```python
from build123d import *
from build123d.topology import SkipClean

# Parameters (mm, degrees)
BOSS_EXTRUDE1_DEPTH           = 2
BOSS_EXTRUDE2_DEPTH           = 80
SKETCH3_R                     = 2.5
BOSS_EXTRUDE3_DEPTH           = 8
BOSS_EXTRUDE3_DRAFT           = 3
BOSS_EXTRUDE3_PROFILE_2_DEPTH = 8
BOSS_EXTRUDE3_PROFILE_2_DRAFT = 3
SHELL2_START                  = 1
SHELL2_OUTLINE_R              = 9
SHELL2_DEPTH                  = 80
CUT_EXTRUDE1_DEPTH            = 93.332280474
BOSS_EXTRUDE4_DEPTH           = 5
BOSS_EXTRUDE5_DEPTH           = 5


with BuildPart() as part:
    # Sketch1 → Boss-Extrude1 (new body)
    with BuildSketch(Plane(origin=(0, 0, 0), x_dir=(1, 0, 0), z_dir=(0, 1, 0))):
        with BuildLine():
            Line((-15, -12.5), (15, -12.5))
            ThreePointArc((15, -12.5), (22.071067812, -9.571067812), (25, -2.5))
            Line((25, -2.5), (25, 2.5))
            ThreePointArc((25, 2.5), (22.071067812, 9.571067812), (15, 12.5))
            Line((15, 12.5), (-15, 12.5))
            ThreePointArc((-15, 12.5), (-22.071067812, 9.571067812), (-25, 2.5))
            Line((-25, 2.5), (-25, -2.5))
            ThreePointArc((-25, -2.5), (-22.071067812, -9.571067812), (-15, -12.5))
        make_face()
    extrude(amount=BOSS_EXTRUDE1_DEPTH)

    # Sketch2 → Boss-Extrude2 (add)
    with BuildSketch(Plane(origin=(0, 2, 0), x_dir=(1, 0, 0), z_dir=(0, 1, 0))):
        with BuildLine():
            ThreePointArc((-20, 0), (-11, 9), (-2, 0))
            Line((-2, 0), (-1, 0))
            ThreePointArc((-1, 0), (-11, 10), (-21, 0))
            Line((-21, 0), (-20, 0))
        make_face()
        with BuildLine():
            Line((-1, 0), (-2, 0))
            ThreePointArc((-2, 0), (-11, -9), (-20, 0))
            Line((-20, 0), (-21, 0))
            ThreePointArc((-21, 0), (-11, -10), (-1, 0))
        make_face()
        with BuildLine():
            ThreePointArc((21, 0), (11, 10), (1, 0))
            Line((1, 0), (2, 0))
            ThreePointArc((2, 0), (11, 9), (20, 0))
            Line((20, 0), (21, 0))
        make_face()
        with BuildLine():
            Line((2, 0), (1, 0))
            ThreePointArc((1, 0), (11, -10), (21, 0))
            Line((21, 0), (20, 0))
            ThreePointArc((20, 0), (11, -9), (2, 0))
        make_face()
        with BuildLine():
            ThreePointArc((20, 0), (11, 9), (2, 0))
            Line((2, 0), (20, 0))
        make_face()
        with BuildLine():
            Line((20, 0), (2, 0))
            ThreePointArc((2, 0), (11, -9), (20, 0))
        make_face()
        with BuildLine():
            ThreePointArc((-20, 0), (-11, -9), (-2, 0))
            Line((-2, 0), (-20, 0))
        make_face()
        with BuildLine():
            Line((-20, 0), (-2, 0))
            ThreePointArc((-2, 0), (-11, 9), (-20, 0))
        make_face()
    extrude(amount=BOSS_EXTRUDE2_DEPTH)


with BuildPart() as boss_extrude3_tool:
    # Sketch3 → Boss-Extrude3 (with draft: the straight prism first)
    with BuildSketch(Plane(origin=(0, 82, 0), x_dir=(1, 0, 0), z_dir=(0, 1, 0))):
        with Locations((-5, 0)):
            Circle(SKETCH3_R)
    extrude(amount=BOSS_EXTRUDE3_DEPTH)
    # Boss-Extrude3: the draft: its side faces are tilted about the plane it starts from
    boss_extrude3_sides = [boss_extrude3_tool.faces().sort_by_distance(p)[0] for p in [
        (-7.5, 86, 0),
    ]]
    draft(boss_extrude3_sides, Plane(origin=(0, 82, 0), x_dir=(1, 0, 0), z_dir=(0, 1, 0)), BOSS_EXTRUDE3_DRAFT)


with BuildPart() as part_1:
    add(part.part)

    # Boss-Extrude3: add boss_extrude3_tool
    add(boss_extrude3_tool.part)


with BuildPart() as boss_extrude3_profile_2_tool:
    # Sketch3 → Boss-Extrude3 profile 2 (with draft: the straight prism first)
    with BuildSketch(Plane(origin=(0, 82, 0), x_dir=(1, 0, 0), z_dir=(0, 1, 0))):
        with Locations((5, 0)):
            Circle(SKETCH3_R)
    extrude(amount=BOSS_EXTRUDE3_PROFILE_2_DEPTH)
    # Boss-Extrude3 profile 2: the draft: its side faces are tilted about the plane it starts from
    boss_extrude3_profile_2_sides = [boss_extrude3_profile_2_tool.faces().sort_by_distance(p)[0] for p in [
        (2.5, 86, 0),
    ]]
    draft(boss_extrude3_profile_2_sides, Plane(origin=(0, 82, 0), x_dir=(1, 0, 0), z_dir=(0, 1, 0)), BOSS_EXTRUDE3_PROFILE_2_DRAFT)


with BuildPart() as part_2:
    add(part_1.part)

    # Boss-Extrude3 profile 2: add boss_extrude3_profile_2_tool
    add(boss_extrude3_profile_2_tool.part)

    # Shell2: read off the stored shape, not the designer's step
    # Shell2 outline → Shell2 (cut)
    with BuildSketch(Plane(origin=(0, 0, 0), x_dir=(1, 0, 0), z_dir=(0, 1, 0)).offset(SHELL2_START)):
        with Locations((11, 0)):
            Circle(SHELL2_OUTLINE_R)
        with Locations((-11, 0)):
            Circle(SHELL2_OUTLINE_R)
    extrude(amount=SHELL2_DEPTH, mode=Mode.SUBTRACT)

    # Shell2 2: loft between two sections, ruled curve by curve
    shell2_2_from = [
        Edge.make_three_point_arc((5, 90, 1.07936542), (3.92063458, 90, 0), (5, 90, -1.07936542)),
        Edge.make_three_point_arc((5, 90, -1.07936542), (6.07936542, 90, 0), (5, 90, 1.07936542)),
    ]
    shell2_2_to = [
        Edge.make_three_point_arc((5, 81, 1.551035433), (3.448964567, 81, 0), (5, 81, -1.551035433)),
        Edge.make_three_point_arc((5, 81, -1.551035433), (6.551035433, 81, 0), (5, 81, 1.551035433)),
    ]
    shell2_2 = Solid(Shell([*[Face.make_surface_from_curves(shell2_2_from[k], shell2_2_to[k]) for k in range(2)], Face(Wire(shell2_2_from)), Face(Wire(shell2_2_to))]))
    add(shell2_2, mode=Mode.SUBTRACT)

    # Shell2 3: loft between two sections, ruled curve by curve
    shell2_3_from = [
        Edge.make_three_point_arc((-5, 90, 1.07936542), (-6.07936542, 90, 0), (-5, 90, -1.07936542)),
        Edge.make_three_point_arc((-5, 90, -1.07936542), (-3.92063458, 90, 0), (-5, 90, 1.07936542)),
    ]
    shell2_3_to = [
        Edge.make_three_point_arc((-5, 81, 1.551035433), (-6.551035433, 81, 0), (-5, 81, -1.551035433)),
        Edge.make_three_point_arc((-5, 81, -1.551035433), (-3.448964567, 81, 0), (-5, 81, 1.551035433)),
    ]
    shell2_3 = Solid(Shell([*[Face.make_surface_from_curves(shell2_3_from[k], shell2_3_to[k]) for k in range(2)], Face(Wire(shell2_3_from)), Face(Wire(shell2_3_to))]))
    add(shell2_3, mode=Mode.SUBTRACT)

    # Sketch2<3> → Cut-Extrude1 (cut, through all)
    with SkipClean():  # the faces are left unmerged after this step: merging them gives an invalid solid
        with BuildSketch(Plane(origin=(0, 2, 0), x_dir=(1, 0, 0), z_dir=(0, 1, 0))):
            with BuildLine():
                ThreePointArc((-20, 0), (-11, -9), (-2, 0))
                Line((-2, 0), (-20, 0))
            make_face()
            with BuildLine():
                Line((-20, 0), (-2, 0))
                ThreePointArc((-2, 0), (-11, 9), (-20, 0))
            make_face()
            with BuildLine():
                ThreePointArc((20, 0), (11, 9), (2, 0))
                Line((2, 0), (20, 0))
            make_face()
            with BuildLine():
                Line((20, 0), (2, 0))
                ThreePointArc((2, 0), (11, -9), (20, 0))
            make_face()
        extrude(amount=-CUT_EXTRUDE1_DEPTH, mode=Mode.SUBTRACT)

    # Sketch4 → Boss-Extrude4 (add, symmetric)
    with SkipClean():  # the faces are left unmerged after this step: merging them gives an invalid solid
        with BuildSketch(Plane(origin=(0, 20, 0), x_dir=(1, 0, 0), z_dir=(0, 1, 0))):
            with BuildLine():
                Line((1, 0), (-1, 0))
                ThreePointArc((-1, 0), (-1.079703037, -1.260042925), (-1.317541634, -2.5))
                Line((-1.317541634, -2.5), (1.317541634, -2.5))
                ThreePointArc((1.317541634, -2.5), (1.079703037, -1.260042925), (1, 0))
            make_face()
            with BuildLine():
                ThreePointArc((-1.317541634, 2.5), (-1.079703037, 1.260042925), (-1, 0))
                Line((-1, 0), (1, 0))
                ThreePointArc((1, 0), (1.079703037, 1.260042925), (1.317541634, 2.5))
                Line((1.317541634, 2.5), (-1.317541634, 2.5))
            make_face()
        extrude(amount=BOSS_EXTRUDE4_DEPTH, both=True)

    # Sketch7 → Boss-Extrude5 (add, symmetric)
    with SkipClean():  # the faces are left unmerged after this step: merging them gives an invalid solid
        with BuildSketch(Plane(origin=(0, 70, 0), x_dir=(1, 0, 0), z_dir=(0, 1, 0))):
            with BuildLine():
                ThreePointArc((-1.317541634, 2.5), (-1.079703037, 1.260042925), (-1, 0))
                Line((-1, 0), (1, 0))
                ThreePointArc((1, 0), (1.079703037, 1.260042925), (1.317541634, 2.5))
                Line((1.317541634, 2.5), (-1.317541634, 2.5))
            make_face()
            with BuildLine():
                Line((1, 0), (-1, 0))
                ThreePointArc((-1, 0), (-1.079703037, -1.260042925), (-1.317541634, -2.5))
                Line((-1.317541634, -2.5), (1.317541634, -2.5))
                ThreePointArc((1.317541634, -2.5), (1.079703037, -1.260042925), (1, 0))
            make_face()
        extrude(amount=BOSS_EXTRUDE5_DEPTH, both=True)


solid = part_2.part
```
Design review of the part built by this model. Coordinates are the model's own, in mm. A direction names the side the tool comes from. Give positions to 0.01 mm unless a question says otherwise; leave off trailing zeros. Loops run counter-clockwise (first coordinate to the right, second up) from the corner with the lowest first, then second, coordinate; pieces in that order, holes last. Notation, with made-up numbers: (40.5, -36) -> (48.5, -36) arc R17 ccw to (48.5, -25) -> close; hole circle Ø6 at (11.5, 66). An arc over 180 degrees is marked (long way). Write each question's results on one line, items separated by ' | '.
Q1. Wall thickness on L1, parallel to Z at x = -11, y = 43; L2, parallel to X at y = 35, z = -6.5; L3, parallel to X at y = 7, z = -4: over which ranges is each line inside the solid? List them lowest first.
Reply:
L1: z = -10 to -9, 9 to 10 | L2: x = -18.6 to -17.22, -4.78 to -3.4, 3.4 to 4.78, 17.22 to 18.6 | L3: x = -20.17 to -19.06, -2.94 to -1.83, 1.83 to 2.94, 19.06 to 20.17
Q2. Take a section at B-B, the plane y = 66.5. Write out the cut boundary in (x, z).
Reply:
outline: (-1.32, -2.5) -> (1.32, -2.5) arc R10 ccw (long way) to (1.32, 2.5) -> (-1.32, 2.5) arc R10 ccw (long way) to start; hole circle Ø18 at (-11, 0); hole circle Ø18 at (11, 0)
Q3. Machinability: for faces 5 (the face through (11, 81, 0)), 6 (the face through (0, 20, -2.5)), 7 (the face through (22.15, 0.99, -9.49)), which of the approach directions +Z, -Z, +X, -X, +Y, -Y give a long, thin tool a straight path to every point of the face, cutting with its end or side? Answer none if there is none.
Reply:
face 5: -Y | face 6: -Z, +Y | face 7: -Z, +X, +Y, -Y
Q4. For pin 1 Ø6 at (y, z) = (23, -1.5) entering from +X; pin 2 Ø3 at (x, z) = (0.5, -1.5) entering from +Y; pin 3 Ø3 at (x, y) = (0.5, 17) entering from +Z, all flat-tipped, find the tip position at first contact; note any pin that passes through.
Reply:
pin 1: stops at x = 21 | pin 2: stops at y = 82 | pin 3: stops at z = 4.36
Q5. Take a section at D-D, the plane z = -5.5. Write out the cut boundary in (x, y).
Reply:
outline: (-24.54, 0) -> (-18.12, 0) -> (-18.12, 81) -> (-3.88, 81) -> (-3.88, 0) -> (3.88, 0) -> (3.88, 81) -> (18.12, 81) -> (18.12, 0) -> (24.54, 0) -> (24.54, 2) -> (19.35, 2) -> (19.35, 82) -> (2.65, 82) -> (2.65, 2) -> (-2.65, 2) -> (-2.65, 82) -> (-19.35, 82) -> (-19.35, 2) -> (-24.54, 2) -> close
Q6. Take a section at A-A, the plane x = 11. Write out the cut boundary in (y, z).
Reply:
outline: (0, -12.5) -> (2, -12.5) -> (2, -10) -> (82, -10) -> (82, 10) -> (2, 10) -> (2, 12.5) -> (0, 12.5) -> (0, 9) -> (81, 9) -> (81, -9) -> (0, -9) -> close
Q7. The part is to be moulded in two halves that separate along X. For faces 1 (the face through (6, 90, 1)), 2 (the face through (-20.54, 41.44, 3)), 3 (the face through (-22.15, 0.99, 9.49)), 4 (the face through (-11, 81, 0)), say which applies: +X half, -X half, draft (parallel to the pull), parting line (faces both ways), or undercut.
Reply:
face 1: draft | face 2: undercut | face 3: -X half | face 4: undercut
Q8. Take a section at C-C, the plane y = 51.5. Write out the cut boundary in (x, z), plus the area to 3 significant figures.
Reply:
outline: circle Ø20 at (-11, 0); circle Ø20 at (11, 0); hole circle Ø18 at (-11, 0); hole circle Ø18 at (11, 0) | area: 119 mm²
